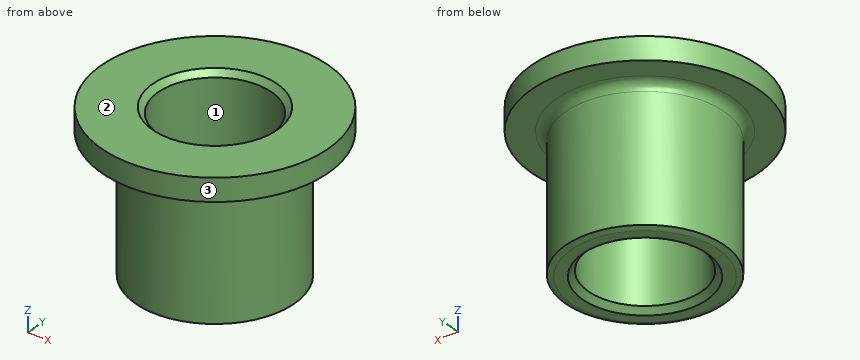
from build123d import *

# Parameters (mm, degrees)
SKETCH_4_R          = 3.5
EXTRUDE_1_DEPTH     = 6
SKETCH_5_R          = 5
EXTRUDE_2_DEPTH     = 1
SKETCH_6_R          = 2.5
CUT_EXTRUDE_1_DEPTH = 8
FILLET_1_R          = 0.4
CHAMFER_1_SIZE      = 0.25
CHAMFER_1_SIZE2     = 0.090992559
CHAMFER_2_SIZE      = 0.25
CHAMFER_3_SIZE      = 0.25


with BuildPart() as part:
    # Эскиз4 → Бобышка-Вытянуть1 (new body)
    with BuildSketch(Plane.XY):
        Circle(SKETCH_4_R)
    extrude(amount=EXTRUDE_1_DEPTH)

    # Эскиз5 → Бобышка-Вытянуть2 (add)
    with BuildSketch(Plane.XY.offset(6)):
        Circle(SKETCH_5_R)
    extrude(amount=EXTRUDE_2_DEPTH)

    # Эскиз6 → Вырез-Вытянуть1 (cut, through all)
    with BuildSketch(Plane.XY.offset(7)):
        Circle(SKETCH_6_R)
    extrude(amount=-CUT_EXTRUDE_1_DEPTH, mode=Mode.SUBTRACT)

    # Скругление1
    fillet_1_edges = [part.edges().sort_by_distance(p)[0] for p in [
        (-3.5, 0, 6),
    ]]
    fillet(fillet_1_edges, radius=FILLET_1_R)

    # Фаска1
    chamfer_1_edges = [part.edges().sort_by_distance(p)[0] for p in [
        (-3.5, 0, 0),
    ]]
    chamfer_1_side = [part.faces().sort_by_distance(p)[0] for p in [
        (-3.401005051, 0, 0),
    ]]
    chamfer(chamfer_1_edges, length=CHAMFER_1_SIZE, length2=CHAMFER_1_SIZE2, reference=chamfer_1_side[0])

    # Фаска2
    chamfer_2_edges = [part.edges().sort_by_distance(p)[0] for p in [
        (-2.5, 0, 0),
    ]]
    chamfer(chamfer_2_edges, length=CHAMFER_2_SIZE)

    # Фаска3
    chamfer_3_edges = [part.edges().sort_by_distance(p)[0] for p in [
        (-2.5, 0, 7),
    ]]
    chamfer(chamfer_3_edges, length=CHAMFER_3_SIZE)


solid = part.part
CAD build for the part. Positions are in the model's coordinates, mm. Face numbers are marked on the shaded views. Round coordinates to 2 decimals unless told otherwise and drop trailing zeros. Order: outer loops, then holes, each group sorted by start corner. A loop starts at its lowest first (then second) coordinate and runs counter-clockwise, first axis right, second up. Notation, with made-up numbers: (-20.5, -3.5) -> (15.5, -3.5) arc R13 ccw to (15.5, 17.5) -> close; hole circle Ø11 at (25, -11.75). An arc over 180 degrees is marked (long way). Write each question's results on one line, items separated by ' | '.
1. Flat gauge pins, fed straight in: P1, Ø3, axis at y = -2.5, z = 3.5, coming from the +X side; P2, Ø4, axis at y = 0.5, z = 2, coming from the -X side; P3, Ø1.5, axis at y = -2, z = 4, coming from the -X side. Where does each tip first touch, or does it go through?
Findings below:
P1: stops at x = 3.35 | P2: stops at x = -3.5 | P3: stops at x = -3.27
2. Wall check: line 1 along Y through (x, z) = (0, 4.5); line 2 along Y through (x, z) = (-0.75, 6.25); line 3 along Z through (x, y) = (3.25, 2.75). Give the ranges that are in metal, low to high. Write a range as [from, to].
Findings below:
line 1: y = [-3.5, -2.5], [2.5, 3.5] | line 2: y = [-4.94, -2.38], [2.38, 4.94] | line 3: z = [6, 7]
3. Pull direction X, two halves, no side cores. Call the marked faces 1, 2 and 3: pulls with the +X half, pulls with the -X half, needs draft (parallel to the pull), parting line crosses it, or undercut.
Findings below:
face 1: undercut | face 2: needs draft | face 3: parting line crosses it
4. Cut at A-A (y = 0). Give the cut face in (x, z).
Findings below:
outline: (-5, 6) -> (-3.9, 6) arc R0.4 cw to (-3.5, 5.6) -> (-3.5, 0.09) -> (-3.25, 0) -> (-2.75, 0) -> (-2.5, 0.25) -> (-2.5, 6.75) -> (-2.75, 7) -> (-5, 7) -> close; (2.5, 0.25) -> (2.75, 0) -> (3.25, 0) -> (3.5, 0.09) -> (3.5, 5.6) arc R0.4 cw to (3.9, 6) -> (5, 6) -> (5, 7) -> (2.75, 7) -> (2.5, 6.75) -> close
5. Cut at C-C (z = 1.25). Give the cut face in (x, y), plus the area to 3 significant figures.
Findings below:
outline: circle Ø7 at (0, 0); hole circle Ø5 at (0, 0) | area: 18.8 mm²
